Source: CAD feature listing. Evaluate the final solid. Frame: model axes, mm. Face numbers are marked on the shaded views. A direction names the side the tool comes from. Coordinates: 2 decimals unless noted, no trailing zeros. Loops run counter-clockwise (first coordinate to the right, second up) from the corner with the lowest first, then second, coordinate; pieces in that order, holes last.
Item 1: Pin query (flat end, axial travel): pin 1 Ø1 at (x, y) = (25, -7) entering from -Z; pin 2 Ø8 at (x, z) = (8, 0) entering from +Y (3 decimals); pin 3 Ø1.5 at (x, z) = (7, 9) entering from +Y; pin 4 Ø5 at (x, z) = (18.5, -2.5) entering from -Y. Return the tip coordinate at first contact, or that it passes through.
Item 2: Section query B-B, the plane x = 18.5. Return the cut outline in (y, z), then the cut area to 3 significant figures.
Item 3: Pull-direction query (Z, two-part tool) for the marked faces 1, 2 and 3; classes: +Z half, -Z half, draft (parallel to the pull), parting line (faces both ways), or undercut.
Item 4: Reachability of the marked faces 4, 5 and 6 from +Z, -Z, +X, -X, +Y, -Y: full face, straight path, thin tool, end or side. Return the list, or none.
Item 5: Line query: probe 1 along Y at (x, z) = (14, 0); probe 2 along Y at (x, z) = (26, 0). Output: solid intervals per line, ascending.
Item 6: Section query A-A, the plane x = 32. Return the cut outline in (y, z), then the cut area to 3 significant figures.
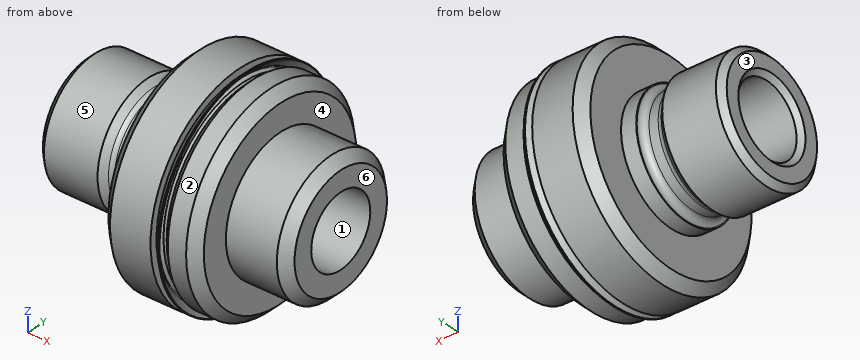
```python
from build123d import *

# Parameters (mm, degrees)
HOLE1_D           = 11.2268
HOLE1_DEPTH       = 39.6748
HOLE1_CSINK_D     = 12.7508
HOLE1_CSINK_ANGLE = 90


with BuildPart() as part:
    # Sketch1 → Revolve1 (revolve)
    with BuildSketch(Plane.XY):
        with BuildLine():
            Line((0, 0), (0, 8.58901))
            Line((0, 8.58901), (0.93599, 9.525))
            Line((0.93599, 9.525), (9.35648951, 9.525))
            Line((9.35648951, 9.525), (10.295571935, 8.59395034))
            ThreePointArc((10.295571935, 8.59395034), (10.624110429, 8.375955547), (11.0109, 8.29945))
            Line((11.0109, 8.29945), (12.446, 8.29945))
            ThreePointArc((12.446, 8.29945), (13.16442049, 8.59702951), (13.462, 9.31545))
            Line((13.462, 9.31545), (13.462, 9.49325))
            Line((13.462, 9.49325), (15.8496, 9.49325))
            Line((15.8496, 9.49325), (15.8496, 0))
            Line((15.8496, 0), (0, 0))
        make_face()
    revolve(axis=Axis((15.8496, 0, 0), (-1, 0, 0)))

    # Sketch2 → Revolve2 (revolve)
    with BuildSketch(Plane.XY):
        Polygon((15.8496, 0), (15.8496, 15.32255), (17.3736, 16.84655), (23.7236, 16.84655), (23.7236, 15.00505), (24.7396, 15.00505), (25.7556, 16.02105), (28.6258, 16.02105), (30.1498, 14.49705), (30.1498, 0), align=None)
    revolve(axis=Axis((30.1498, 0, 0), (-1, 0, 0)))

    # Sketch3 → Revolve3 (revolve)
    with BuildSketch(Plane.XY):
        Polygon((30.1498, 0), (30.1498, 10.3124), (38.1508, 10.3124), (39.6748, 8.7884), (39.6748, 0), align=None)
    revolve(axis=Axis((39.6748, 0, 0), (-1, 0, 0)))

    # Hole1
    with Locations(Plane.ZY):
        with Locations((0, 0)):
            CounterSinkHole(HOLE1_D / 2, HOLE1_CSINK_D / 2, depth=HOLE1_DEPTH, counter_sink_angle=HOLE1_CSINK_ANGLE)

    # Sketch6 → Revolve4 (revolve)
    with BuildSketch(Plane.XY):
        with BuildLine():
            Line((23.7236, 14.75105), (24.7396, 14.75105))
            Line((24.7396, 14.75105), (24.7396, 15.00505))
            Line((24.7396, 15.00505), (24.2316, 15.00505))
            Line((24.2316, 15.00505), (23.856982072, 15.379667928))
            ThreePointArc((23.856982072, 15.379667928), (23.819784633, 15.46947049), (23.856982072, 15.559273051))
            Line((23.856982072, 15.559273051), (25.060090825, 16.762381804))
            Line((25.060090825, 16.762381804), (25.060090825, 16.84655))
            Line((25.060090825, 16.84655), (24.856890825, 16.84655))
            Line((24.856890825, 16.84655), (23.7236, 15.713259175))
            Line((23.7236, 15.713259175), (23.7236, 14.75105))
        make_face()
    revolve(axis=Axis((24.7396, 0, 0), (-1, 0, 0)))


solid = part.part
```
Verdict:
1. pin 1: stops at z = -15.54
1. pin 2: stops at y = 9.525
1. pin 3: stops at y = 4.76
1. pin 4: stops at y = -16.85
2. outline: circle Ø33.69 at (0, 0); hole circle Ø11.23 at (0, 0)
2. area: 793 mm2
3. face 1: undercut
3. face 2: parting line
3. face 3: draft
4. face 4: +X
4. face 5: -X
4. face 6: +Z, -Z, +X, +Y, -Y
5. probe 1: y = -9.49 to -5.61, 5.61 to 9.49
5. probe 2: y = -16.02 to -5.61, 5.61 to 16.02
6. outline: circle Ø20.62 at (0, 0); hole circle Ø11.23 at (0, 0)
6. area: 235 mm2
